Geometry: final body of the model. Coordinates: model frame, mm. Give positions to 0.01 mm unless a question says otherwise; leave off trailing zeros. Order: outer loops, then holes, each group sorted by start corner. A loop starts at its lowest first (then second) coordinate and runs counter-clockwise, first axis right, second up. Notation, with made-up numbers: (80, -14) - (128, -14) arc R23 cw to (128, 4) - close; hole circle Ø10 at (78, -13.75). An arc over 180 degrees is marked (long way). Put each result on its own line as item: value. Start each with the question number.
1. Section A-A on y = -96.5. Return the cut outline in (x, z), plus the area to 3 significant figures.
2. Section B-B on z = 0.7. Return the cut outline in (x, y), plus the area to 3 significant figures.
3. First-contact query: P1, Ø0.6, axis at x = -170, z = 1.5, coming from the -Y side; P2, Ø0.6, axis at y = -261, z = 1, coming from the -X side; P3, Ø10, axis at x = -131, y = -204, coming from the -Z side; P4, Ø0.6, axis at x = 172.5, z = 1.5, coming from the -Y side. Flat tips, straight axial feed; report the tip coordinate or a pass-through.
4. Section D-D on x = 113. Return the cut outline in (y, z), plus the area to 3 significant figures.
5. Section C-C on y = -245. Return the cut outline in (x, z).
6. Ray query, line 1 along X through (y, z) = (-87.5, 1.4); line 2 along Y through (x, z) = (115, 1.6); line 3 along Y through (x, z) = (181, 1.45). Return the intervals inside material, ascending. Write a range as from..to.
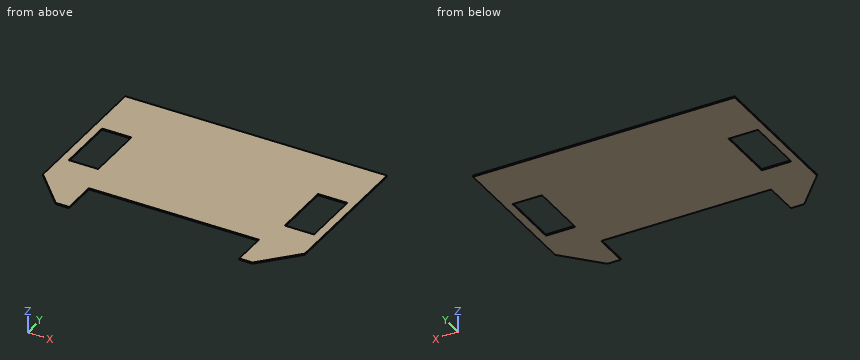
from build123d import *

# Parameters (mm, degrees)
SKETCH1_W           = 45
SKETCH1_H           = 90
BOSS_EXTRUDE1_DEPTH = 2


with BuildPart() as part:
    # Sketch1 → Boss-Extrude1 (new body)
    with BuildSketch(Plane.XY):
        Polygon((200, 0), (-200, 0), (-200, -222.5), (-150.404334867, -275.82), (-130, -275.82), (-130, -222.5), (130, -222.5), (130, -275.82), (150.404334867, -275.82), (200, -222.5), align=None)
        with Locations((-165, -130)):
            Rectangle(SKETCH1_W, SKETCH1_H, mode=Mode.SUBTRACT)
        with Locations((165, -130)):
            Rectangle(SKETCH1_W, SKETCH1_H, mode=Mode.SUBTRACT)
    extrude(amount=BOSS_EXTRUDE1_DEPTH)


solid = part.part
Resolved:
1. outline: (-200, 0) - (-187.5, 0) - (-187.5, 2) - (-200, 2) - close; (-142.5, 0) - (142.5, 0) - (142.5, 2) - (-142.5, 2) - close; (187.5, 0) - (200, 0) - (200, 2) - (187.5, 2) - close
1. area: 620 mm^2
2. outline: (-200, -222.5) - (-150.4, -275.82) - (-130, -275.82) - (-130, -222.5) - (130, -222.5) - (130, -275.82) - (150.4, -275.82) - (200, -222.5) - (200, 0) - (-200, 0) - close; hole (-187.5, -175) - (-142.5, -175) - (-142.5, -85) - (-187.5, -85) - close; hole (142.5, -175) - (187.5, -175) - (187.5, -85) - (142.5, -85) - close
2. area: 85,700 mm^2
3. P1: y = -255.08
3. P2: x = -164.47
3. P3: z = 0
3. P4: y = -252.39
4. outline: (-222.5, 0) - (0, 0) - (0, 2) - (-222.5, 2) - close
4. area: 445 mm^2
5. outline: (-179.07, 0) - (-130, 0) - (-130, 2) - (-179.07, 2) - close; (130, 0) - (179.07, 0) - (179.07, 2) - (130, 2) - close
6. line 1: -200..-187.5, -142.5..142.5, 187.5..200
6. line 2: -222.5..0
6. line 3: -242.93..-175, -85..0
